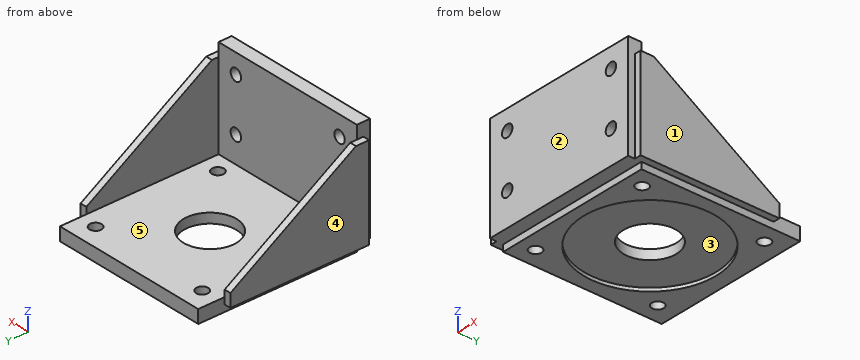
from build123d import *

# Parameters (mm, degrees)
SKETCH1_W                 = 152.4
SKETCH1_H                 = 152.4
BASE_EXTRUDE_DEPTH        = 12.7
SKETCH2_W                 = 101.6
SKETCH2_H                 = 12.7
BOSS_EXTRUDE1_DEPTH       = 152.4
BOSS_EXTRUDE2_DEPTH       = 6.35
SKETCH5_R                 = 63.5635
PILOT_BORE_DEPTH          = 3.302
SKETCH6_R                 = 25.4
CUT_EXTRUDE3_DEPTH        = 160.339822581
SKETCH_PATTERN1_OUTLINE_R = 5.75437
SKETCH_PATTERN1_DEPTH     = 12.7
LPATTERN1_COUNT           = 2
LPATTERN1_PITCH           = 114.3
LPATTERN1_COUNT_DIR2      = 2
LPATTERN1_PITCH_DIR2      = 50.8


# Read off the part's stored shape, not the designer's step: Sketch-Pattern1
with BuildPart() as part:
    # Sketch1 → Base-Extrude (new body)
    with BuildSketch(Plane.XY):
        with Locations((0, 1.5875)):
            Rectangle(SKETCH1_W, SKETCH1_H)
    extrude(amount=BASE_EXTRUDE_DEPTH)

    # Sketch2 → Boss-Extrude1 (add)
    with BuildSketch(Plane(origin=(76.2, 0, 0), x_dir=(0, 0, -1), z_dir=(1, 0, 0))):
        with Locations((-57.15, -80.9625)):
            Rectangle(SKETCH2_W, SKETCH2_H)
    extrude(amount=-BOSS_EXTRUDE1_DEPTH)

    # Sketch3 → Boss-Extrude2 (add)
    with BuildSketch(Plane(origin=(76.2, 0, 0), x_dir=(0, 0, -1), z_dir=(1, 0, 0))):
        Polygon((-6.35, -80.9625), (-6.35, 52.3875), (-19.05, 52.3875), (-95.25, -68.2625), (-95.25, -80.9625), align=None)
    boss_extrude2 = extrude(amount=BOSS_EXTRUDE2_DEPTH)

    # Mirror1: Boss-Extrude2 across plane
    add(boss_extrude2.mirror(Plane(origin=(0, 0, 0), x_dir=(0, 0, 1), z_dir=(1, 0, 0))))

    # Sketch5 → pilot bore (cut)
    with BuildSketch(Plane(origin=(0, 0, 0), x_dir=(-1, 0, 0), z_dir=(0, 0, -1))):
        Circle(SKETCH5_R)
    extrude(amount=-PILOT_BORE_DEPTH, mode=Mode.SUBTRACT)

    # Sketch6 → Cut-Extrude3 (cut, through all)
    with BuildSketch(Plane(origin=(0, 0, 3.302), x_dir=(-1, 0, 0), z_dir=(0, 0, -1))):
        Circle(SKETCH6_R)
    extrude(amount=-CUT_EXTRUDE3_DEPTH, mode=Mode.SUBTRACT)

    # Sketch7 → 1/2-20 Tapped Hole1 (revolve, cut)
    with BuildSketch(Plane(origin=(-58.7375, -58.7375, 12.7), x_dir=(0, -1, 0), z_dir=(1, 0, 0))):
        Polygon((0, 0), (0, 35.20757432), (5.75437, 31.75), (5.75437, 0), align=None)
    revolve(axis=Axis((-58.7375, -58.7375, 19.05), (0, 0, -1)), mode=Mode.SUBTRACT)

    # Sketch-Pattern1 outline → Sketch-Pattern1 (cut)
    with BuildSketch(Plane.XY):
        with Locations((-58.7375, 58.7375)):
            Circle(SKETCH_PATTERN1_OUTLINE_R)
        with Locations((58.7375, 58.7375)):
            Circle(SKETCH_PATTERN1_OUTLINE_R)
        with Locations((58.7375, -58.7375)):
            Circle(SKETCH_PATTERN1_OUTLINE_R)
    extrude(amount=SKETCH_PATTERN1_DEPTH, mode=Mode.SUBTRACT)

    # Sketch9 → 1/2-20 Tapped Hole2 (revolve, cut)
    with BuildSketch(Plane(origin=(-57.15, -74.6125, 88.9), x_dir=(0, 0, 1), z_dir=(1, 0, 0))):
        Polygon((0, 0), (0, 35.20757432), (5.75437, 31.75), (5.75437, 0), align=None)
    f_1_2_20_tapped_hole2 = revolve(axis=Axis((-57.15, -68.2625, 88.9), (0, -1, 0)), mode=Mode.SUBTRACT)

    # LPattern1: 1_2-20 Tapped Hole2 2 × 2
    with Locations(*[(i * LPATTERN1_PITCH, 0, -j * LPATTERN1_PITCH_DIR2) for i in range(LPATTERN1_COUNT) for j in range(LPATTERN1_COUNT_DIR2) if (i, j) != (0, 0)]):
        add(f_1_2_20_tapped_hole2, mode=Mode.SUBTRACT)


solid = part.part
Work out the finished part from the listing and answer in its coordinate system (mm). Face numbers are marked on the shaded views. A direction names the side the tool comes from. Round coordinates to 2 decimals unless told otherwise and drop trailing zeros. Loops run counter-clockwise (first coordinate to the right, second up) from the corner with the lowest first, then second, coordinate; pieces in that order, holes last. Notation, with made-up numbers: (21, 85) - (61, 85) arc R24 ccw to (61, 122) - close; hole circle Ø3 at (3, 86.25). An arc over 180 degrees is marked (long way). One line per item, written item: value.
Q1. For the marked faces 4 and 5, determine the directions among +Z, -Z, +X, -X, +Y, -Y from which every point of the face is accessible in a straight line to the end or side of a thin tool.
Check values:
face 4: +Z, -Z, -X, +Y, -Y
face 5: +Z, +Y
Q2. Find section D-D on x = -23. Give the vertices of the cut face in (y, z).
Check values:
outline: (-87.31, 6.35) - (-74.61, 6.35) - (-74.61, 0) - (-59.26, 0) - (-59.26, 3.3) - (-10.78, 3.3) - (-10.78, 12.7) - (-74.61, 12.7) - (-74.61, 107.95) - (-87.31, 107.95) - close; (10.78, 3.3) - (59.26, 3.3) - (59.26, 0) - (77.79, 0) - (77.79, 12.7) - (10.78, 12.7) - close
Q3. Straight lines are drawn through the part: probe 1 along Z at (x, y) = (-57.15, -81.5); probe 2 along X at (y, z) = (-77.25, 88.9); probe 3 along X at (y, z) = (-3.5, 47). For each, find the intervals that lie inside material, in ascending order.
Check values:
probe 1: 6.35 to 32.35, 43.85 to 83.15, 94.65 to 107.95
probe 2: -82.55 to -62.9, -51.4 to 51.4, 62.9 to 82.55
probe 3: -82.55 to -76.2, 76.2 to 82.55
Q4. Find section A-A on y = -3.5. Give the vertices of the cut face in (x, z).
Check values:
outline: (-82.55, 6.35) - (-76.2, 6.35) - (-76.2, 0) - (-63.47, 0) - (-63.47, 3.3) - (-25.16, 3.3) - (-25.16, 12.7) - (-76.2, 12.7) - (-76.2, 54.35) - (-82.55, 54.35) - close; (25.16, 3.3) - (63.47, 3.3) - (63.47, 0) - (76.2, 0) - (76.2, 6.35) - (82.55, 6.35) - (82.55, 54.35) - (76.2, 54.35) - (76.2, 12.7) - (25.16, 12.7) - close
Q5. Find section C-C on x = 57.15. Give the vertices of the cut face in (y, z).
Check values:
outline: (-87.31, 6.35) - (-74.61, 6.35) - (-74.61, 0) - (-64.27, 0) - (-64.27, 12.7) - (-74.61, 12.7) - (-74.61, 32.35) - (-87.31, 32.35) - close; (-87.31, 43.85) - (-74.61, 43.85) - (-74.61, 83.15) - (-87.31, 83.15) - close; (-87.31, 94.65) - (-74.61, 94.65) - (-74.61, 107.95) - (-87.31, 107.95) - close; (-53.21, 0) - (-27.82, 0) - (-27.82, 3.3) - (27.82, 3.3) - (27.82, 0) - (53.21, 0) - (53.21, 12.7) - (-53.21, 12.7) - close; (64.27, 0) - (77.79, 0) - (77.79, 12.7) - (64.27, 12.7) - close
Q6. Find section B-B on z = 38.1. State how many separate pieces and enclosed holes the cut face has, and give its area (3 significant figures).
Check values:
separate pieces: 3
enclosed holes: 0
area: 2,950 mm2
Q7. The mould has two halves that part along Y. Classify the marked faces 1, 2 and 3: +Y half, -Y half, draft (parallel to the pull), parting line (faces both ways), or undercut.
Check values:
face 1: draft
face 2: -Y half
face 3: undercut
Q8. Each of these flat-tipped pins is pushed along its axis until it touches: pin 1 Ø2 at (x, z) = (-5.5, 35.5) entering from +Y; pin 2 Ø7 at (x, z) = (57.15, 38.1) entering from +Y; pin 3 Ø3 at (x, y) = (-79, -72) entering from +Z; pin 4 Ø6 at (y, z) = (56.5, 14.5) entering from +X. Where does it stop, or does it pass through?
Check values:
pin 1: y = -74.61
pin 2: through
pin 3: z = 95.25
pin 4: x = 76.2
